Check sheet for the modelled part. Datum: model origin and axes. Units: mm. Face numbers are marked on the shaded views. A direction names the side the tool comes from. Round coordinates to 2 decimals unless told otherwise and drop trailing zeros. Order: outer loops, then holes, each group sorted by start corner. A loop starts at its lowest first (then second) coordinate and runs counter-clockwise, first axis right, second up.
(1) Sectioned sample at A-A, the plane y = 7.5. Enter the section's corners in (x, z).
(2) Sectioned sample at D-D, the plane y = 83. Enter the section's corners in (x, z), and give its area (3 significant figures).
(3) Sectioned sample at C-C, the plane z = 15. Enter the section's corners in (x, y), and give its area (3 significant figures).
(4) Mould release check, pull along X, two halves, no side actions. Record for the marked faces 1 and 2: released by +X, released by -X, zero draft, split by the parting line, or undercut.
(5) Sectioned sample at B-B, the plane x = -7.5. Enter the section's corners in (y, z).
(6) Thickness scan on probe 1 along Z at (x, y) = (-6.5, 43); probe 2 along X at (y, z) = (63, 1); probe 3 along X at (y, z) = (200.5, 21.35). Record the ranges inside material, lowest first.
(7) Depth check by flat-ended pin: pin 1 (3 mm diameter, centred on x = -35.51, y = 7.5, fed in from -Z); pin 2 (10 mm diameter, centred on y = 28.5, z = -11.5, fed in from -X). Enter the tip coordinate at first touch or a pass-through.
(8) Tool access check on the marked faces 3 and 4. Record the directions out of +Z, -Z, +X, -X, +Y, -Y that give a thin tool (end or side, any length) a straight path to the whole face; none if there is none.
```python
from build123d import *

# Parameters (mm, degrees)
BOSS_EXTRUDE1_DEPTH = 208
SKETCH3_R           = 2.5
CUT_EXTRUDE1_DEPTH  = 60


with BuildPart() as part:
    # Sketch2 → Boss-Extrude1 (new body)
    with BuildSketch(Plane(origin=(0, 0, 0), x_dir=(1, 0, 0), z_dir=(0, 1, 0))):
        with BuildLine():
            Line((-45.279686395, -20), (-40.311288741, -20))
            ThreePointArc((-40.311288741, -20), (-45, 0), (-40.311288741, 20))
            Line((-40.311288741, 20), (-45.279686395, 20))
            ThreePointArc((-45.279686395, 20), (-49.5, 0), (-45.279686395, -20))
        make_face()
        with BuildLine():
            ThreePointArc((45, 0), (43.812144397, -10.271124735), (40.311288741, -20))
            Line((40.311288741, -20), (45.279686395, -20))
            ThreePointArc((45.279686395, -20), (48.433430998, -10.22021339), (49.5, 0))
            ThreePointArc((49.5, 0), (48.433430998, 10.22021339), (45.279686395, 20))
            Line((45.279686395, 20), (40.311288741, 20))
            ThreePointArc((40.311288741, 20), (43.812144397, 10.271124735), (45, 0))
        make_face()
        with BuildLine():
            ThreePointArc((-37.7458607, -24.5), (-39.093377249, -22.286943605), (-40.311288741, -20))
            Line((-40.311288741, -20), (-45.279686395, -20))
            ThreePointArc((-45.279686395, -20), (-44.202957773, -22.278880674), (-43.011626335, -24.5))
            Line((-43.011626335, -24.5), (-37.7458607, -24.5))
        make_face()
        with BuildLine():
            Line((45.279686395, -20), (40.311288741, -20))
            ThreePointArc((40.311288741, -20), (39.093377249, -22.286943605), (37.7458607, -24.5))
            Line((37.7458607, -24.5), (43.011626335, -24.5))
            ThreePointArc((43.011626335, -24.5), (44.202957773, -22.278880674), (45.279686395, -20))
        make_face()
        with BuildLine():
            Line((40.311288741, -20), (0, -20))
            Line((0, -20), (-40.311288741, -20))
            ThreePointArc((-40.311288741, -20), (-39.093377249, -22.286943605), (-37.7458607, -24.5))
            Line((-37.7458607, -24.5), (37.7458607, -24.5))
            ThreePointArc((37.7458607, -24.5), (39.093377249, -22.286943605), (40.311288741, -20))
        make_face()
        with BuildLine():
            Line((-45.279686395, 20), (-40.311288741, 20))
            ThreePointArc((-40.311288741, 20), (-39.093377249, 22.286943605), (-37.7458607, 24.5))
            Line((-37.7458607, 24.5), (-43.011626335, 24.5))
            ThreePointArc((-43.011626335, 24.5), (-44.202957773, 22.278880674), (-45.279686395, 20))
        make_face()
        with BuildLine():
            ThreePointArc((37.7458607, 24.5), (39.093377249, 22.286943605), (40.311288741, 20))
            Line((40.311288741, 20), (45.279686395, 20))
            ThreePointArc((45.279686395, 20), (44.202957773, 22.278880674), (43.011626335, 24.5))
            Line((43.011626335, 24.5), (37.7458607, 24.5))
        make_face()
        with BuildLine():
            Line((-40.311288741, 20), (0, 20))
            Line((0, 20), (40.311288741, 20))
            ThreePointArc((40.311288741, 20), (39.093377249, 22.286943605), (37.7458607, 24.5))
            Line((37.7458607, 24.5), (-37.7458607, 24.5))
            ThreePointArc((-37.7458607, 24.5), (-39.093377249, 22.286943605), (-40.311288741, 20))
        make_face()
    extrude(amount=BOSS_EXTRUDE1_DEPTH)

    # Sketch3 → Cut-Extrude1 (cut)
    with BuildSketch(Plane.XY.offset(24.5)):
        with Locations((-35.511626335, 200.5)):
            Circle(SKETCH3_R)
        with Locations((34.488373665, 200.5)):
            Circle(SKETCH3_R)
        with Locations((34.488373665, 7.5)):
            Circle(SKETCH3_R)
        with Locations((-35.511626335, 7.5)):
            Circle(SKETCH3_R)
    extrude(amount=-CUT_EXTRUDE1_DEPTH, mode=Mode.SUBTRACT)


solid = part.part
```
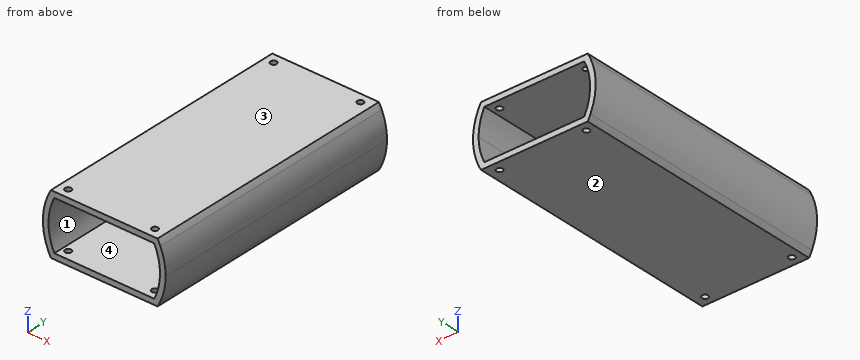
Derived:
1. outline: (-43.01, -24.5) - (-38.01, -24.5) - (-38.01, -20) - (-40.31, -20) arc R45 cw to (-40.31, 20) - (-38.01, 20) - (-38.01, 24.5) - (-43.01, 24.5) arc R49.5 ccw to start; (-33.01, -24.5) - (31.99, -24.5) - (31.99, -20) - (-33.01, -20) - close; (-33.01, 20) - (31.99, 20) - (31.99, 24.5) - (-33.01, 24.5) - close; (36.99, -24.5) - (43.01, -24.5) arc R49.5 ccw to (43.01, 24.5) - (36.99, 24.5) - (36.99, 20) - (40.31, 20) arc R45 cw to (40.31, -20) - (36.99, -20) - close
2. outline: (-43.01, -24.5) - (43.01, -24.5) arc R49.5 ccw to (43.01, 24.5) - (-43.01, 24.5) arc R49.5 ccw to start; hole (-40.31, -20) - (40.31, -20) arc R45 ccw to (40.31, 20) - (-40.31, 20) arc R45 ccw to start
2. area: 1,170 mm2
3. outline: (-47.17, 0) - (-42.43, 0) - (-42.43, 208) - (-47.17, 208) - close; (42.43, 0) - (47.17, 0) - (47.17, 208) - (42.43, 208) - close
3. area: 1,970 mm2
4. face 1: undercut
4. face 2: zero draft
5. outline: (0, -24.5) - (208, -24.5) - (208, -20) - (0, -20) - close; (0, 20) - (208, 20) - (208, 24.5) - (0, 24.5) - close
6. probe 1: z = -24.5 to -20, 20 to 24.5
6. probe 2: x = -49.49 to -44.99, 44.99 to 49.49
6. probe 3: x = -44.66 to -38.01, -33.01 to 31.99, 36.99 to 44.66
7. pin 1: passes through
7. pin 2: stops at x = -49.07
8. face 3: +Z, +X, -X, +Y, -Y
8. face 4: +Y, -Y
